Autodesk Inventor part; units mm, degrees
ref_plane "YZ Plane" through (0, 0, 0) normal (1, 0, 0) x (0, 1, 0)
ref_plane "XZ Plane" through (0, 0, 0) normal (0, 1, 0) x (-1, 0, 0)
ref_plane "XY Plane" through (0, 0, 0) normal (0, 0, 1) x (1, 0, 0)
sketch "Szkic1" plane through (0, 0, 0) normal (0, 0, 1) x (1, 0, 0)
  line L0 (0, 0) -> (20, 0)
  line L1 (20, 0) -> (20, 20)
  line L2 (20, 20) -> (0, 20)
  line L3 (0, 20) -> (0, 0)
  dimension "d0" = 20
  dimension "d1" = 20
extrude "Wyciągnięcie proste1" add sketch "Szkic1" against normal blind 5
sketch "Szkic2" plane through (0, 0, 0) normal (0, 0, 1) x (1, 0, 0)
  line L0 (0, 0) -> (0, 20)
  line L1 (0, 20) -> (0, 5)
  line L2 (0, 5) -> (20, 5)
  line L3 (20, 20) -> (20, 0)
  line L4 (20, 5) -> (20, 20)
  line L5 (0, 20) -> (20, 20)
  line L6 (20, 20) -> (0, 20)
  dimension "d4" = 15
extrude "Wyciągnięcie proste2" add sketch "Szkic2" along normal blind 5
sketch "Szkic3" plane through (0, 0, 5) normal (0, 0, 1) x (1, 0, 0)
  line L0 (0, 20) -> (20, 20)
  line L1 (0, 20) -> (0, -25)
  line L2 (0, -25) -> (20, -25)
  line L3 (20, 20) -> (20, 0)
  line L4 (20, -25) -> (20, 20)
  line L5 (20, 20) -> (0, 20)
  point P0 (0, 0)
  dimension "d7" = 45
extrude "Wyciągnięcie proste3" add sketch "Szkic3" along normal blind 5
sketch "Szkic4" plane through (0, 0, 10) normal (0, 0, 1) x (1, 0, 0)
  line L0 (0, -25) -> (0, -20)
  line L1 (0, 5) -> (0, -25)
  line L2 (0, -20) -> (20, -20)
  line L3 (20, -25) -> (20, 5)
  line L4 (0, -25) -> (20, -25)
  line L5 (20, -25) -> (0, -25)
  point P0 (0, 0)
  dimension "d10" = 5
extrude "Wyciągnięcie proste4" cut sketch "Szkic4" against normal blind 10
sketch "Szkic5" plane through (0, 0, 5) normal (0, 0, -1) x (-1, 0, 0)
  line L0 (0, 20) -> (0, -20)
  line L1 (0, -20) -> (0, -15)
  line L2 (0, -15) -> (-20, -15)
  line L3 (-20, -20) -> (-20, 20)
  line L4 (-20, -20) -> (0, -20)
  point P0 (0, 0)
extrude "Wyciągnięcie proste5" add sketch "Szkic5" along normal blind 5
fillet "Zaokrąglenie1" radius 3 1 edges at (10, -20, 10)
chamfer "Faza1" distance 10 angle 45 1 edges at (10, 20, 10)
fillet "Zaokrąglenie2" radius 5 1 edges at (10, 20, 0)
fillet "Zaokrąglenie3" radius 10 1 edges at (10, 10, 10)
sketch "Szkic6" plane through (0, 0, -5) normal (0, 0, -1) x (-1, 0, 0)
  point P0 (0, 0)
  point P1 (-10.1338, 16.9533)
hole "Otwór1" at (10.1338, 16.9533, -5) direction (0, 0, 1) diameter 3 end through all
properties part number "Otwieracz do butelek"
Part model, mm, in its own coordinate system. A direction names the side the tool comes from. Coordinates: 2 decimals unless noted, no trailing zeros. Order: outer loops, then holes, each group sorted by start corner. A loop starts at its lowest first (then second) coordinate and runs counter-clockwise, first axis right, second up.
(1) Probe L1, parallel to Z at x = 2, y = 1.5; L2, parallel to Y at x = 6.25, z = -2.25; L3, parallel to Z at x = 12.5, y = -11.5. List the from-to ranges inside material, lowest first.
Check sheet entries:
L1: z = -5 to 0, 5 to 10
L2: y = 0 to 20
L3: z = 5 to 10
(2) Slice it at D-D, the plane z = 3. Write the cut outline in (x, y), and give its area (3 significant figures).
Check sheet entries:
outline: (0, -20) - (20, -20) - (20, -15) - (0, -15) - close; (0, 5) - (20, 5) - (20, 17) - (11.63, 17) arc R1.5 cw (long way) to (8.63, 17) - (0, 17) - close
area: 336 mm2
(3) Pull direction X, two halves, no side cores. Call faces 1 (the face through (10.068, 15.455, -1.212)), 2 (the face through (10, -20, 4)), 3 (the face through (20, 0, 6)): pulls with the +X half, pulls with the -X half, needs draft (parallel to the pull), parting line crosses it, or undercut.
Check sheet entries:
face 1: undercut
face 2: needs draft
face 3: pulls with the +X half
(4) Pin check, flat tips, straight feed: pin 1 Ø5.5 at (x, z) = (14, 2.5) entering from +Y; pin 2 Ø4 at (x, z) = (8, -2.5) entering from -Y; pin 3 Ø1.5 at (x, y) = (13, -17) entering from -Z. Stop position of each tip, or through.
Check sheet entries:
pin 1: stops at y = 19.66
pin 2: stops at y = 0
pin 3: stops at z = 0
(5) Slice it at C-C, the plane y = -4. Write the cut outline in (x, z).
Check sheet entries:
outline: (0, 5) - (20, 5) - (20, 10) - (0, 10) - close
(6) Tool access for faces 4 (the face through (10, 0, -2)), 5 (the face through (10, -5, 5)), 6 (the face through (10, -15, 3)), 7 (the face through (10, -5, 10)): list every direction of +Z, -Z, +X, -X, +Y, -Y with a clear straight run to the whole face (end or side of a thin tool).
Check sheet entries:
face 4: -Z, +X, -X, -Y
face 5: +X, -X
face 6: -Z, +X, -X
face 7: +Z, +X, -X, +Y, -Y
(7) Slice it at A-A, the plane z = 0.75. Write the cut outline in (x, y), and give its area (3 significant figures).
Check sheet entries:
outline: (0, -20) - (20, -20) - (20, -15) - (0, -15) - close; (0, 5) - (20, 5) - (20, 19.13) - (0, 19.13) - close; hole circle Ø3 at (10.13, 16.95)
area: 375 mm2
(8) Slice it at B-B, the plane x = 7.25. Write the cut outline in (y, z), and give its area (3 significant figures).
Check sheet entries:
outline: (-20, 0) - (-15, 0) - (-15, 5) - (5, 5) - (5, 0) - (0, 0) - (0, -5) - (20, -5) - (20, -2.07) arc R5 ccw to (18.54, 1.46) - (12.93, 7.07) arc R10 ccw to (5.86, 10) - (-17, 10) arc R3 ccw to (-20, 7) - close
area: 345 mm2
